Read the model definition and answer for the solid it produces. Units are mm, in the model's axes. A direction names the side the tool comes from. Give positions to 0.01 mm unless a question says otherwise; leave off trailing zeros. Order: outer loops, then holes, each group sorted by start corner. A loop starts at its lowest first (then second) coordinate and runs counter-clockwise, first axis right, second up.
```python
from build123d import *

# Parameters (mm, degrees)
F1_DEPTH = 20
F2_W     = 33
F2_H     = 34
F3_DEPTH = 39.001
F4_DEPTH = 6
F5_W     = 7.814886
F5_H     = 15.629771
F6_DEPTH = 25
F7_W     = 19.637413
F7_H     = 8.21565
F8_DEPTH = 39.001


with BuildPart() as f1:
    # F0 (on Front) → F1 (new body, symmetric)
    with BuildSketch(Plane.XZ):
        Polygon((0, 39), (0, 0), (39, 0), (39, 7), (7, 39), align=None)
    extrude(amount=F1_DEPTH, both=True)

    # F2 (on Top) → F3 (cut, through all)
    with BuildSketch(Plane.XY):
        with Locations((22.5, 0)):
            Rectangle(F2_W, F2_H)
    extrude(amount=F3_DEPTH, mode=Mode.SUBTRACT)

    # F2 (on Top) → F4 (join)
    with BuildSketch(Plane.XY):
        with Locations((22.5, 0)):
            Rectangle(F2_W, F2_H)
    extrude(amount=F4_DEPTH)

    # F5 (on face) → F6 (cut)
    with BuildSketch(Plane.YZ.offset(6)):
        with Locations((0, 22.542938)):
            Rectangle(F5_W, F5_H)
    extrude(amount=-F6_DEPTH, mode=Mode.SUBTRACT)

    # F7 (on Top) → F8 (cut, through all)
    with BuildSketch(Plane.XY):
        with Locations((22.542938, 0)):
            Rectangle(F7_W, F7_H)
    extrude(amount=F8_DEPTH, mode=Mode.SUBTRACT)


solid = f1.part
```
1) Given pin 1 (3 mm diameter, centred on y = 1.5, z = 4, fed in from -X); pin 2 (10 mm diameter, centred on x = 20, y = 8, fed in from +Z), each flat-ended and moving along its own axis, determine where each tip first touches the part or whether it passes through.
Final values:
pin 1: stops at x = 0
pin 2: stops at z = 6
2) For a pull along Y with two mould halves and no side action, classify faces 4 (the face through (15, 20, 15)), 5 (the face through (19, 17, 19)), 6 (the face through (15, -20, 15)) as released by +Y, released by -Y, zero draft, split by the parting line, or undercut.
Final values:
face 4: released by +Y
face 5: undercut
face 6: released by -Y
3) A tool of negligible diameter and unlimited length cuts with its end or side. For faces 1 (the face through (3, 0, 14.728)), 2 (the face through (19, -17, 19)), 3 (the face through (22, 4.108, 3)), from which of +Z, -Z, +X, -X, +Y, -Y can it reach the whole face along a straight path? Write none if from no direction.
Final values:
face 1: +X, -X
face 2: +Z, +X
face 3: +Z, -Z
4) The part is cut by section C-C on x = 11.5. Determine the outline of the cut face in (y, z), and give its area (3 significant figures).
Final values:
outline: (-20, 0) - (20, 0) - (20, 34.5) - (17, 34.5) - (17, 6) - (-17, 6) - (-17, 34.5) - (-20, 34.5) - close
area: 411 mm2
5) The part is cut by section A-A on x = 16.5. Determine the outline of the cut face in (y, z), and give its area (3 significant figures).
Final values:
outline: (-20, 0) - (-4.11, 0) - (-4.11, 6) - (-17, 6) - (-17, 29.5) - (-20, 29.5) - close; (4.11, 0) - (20, 0) - (20, 29.5) - (17, 29.5) - (17, 6) - (4.11, 6) - close
area: 332 mm2
6) The part is cut by section D-D on z = 4. Determine the outline of the cut face in (x, y), and give its area (3 significant figures).
Final values:
outline: (0, -20) - (39, -20) - (39, 20) - (0, 20) - close; hole (12.72, -4.11) - (32.36, -4.11) - (32.36, 4.11) - (12.72, 4.11) - close
area: 1,400 mm2
7) The part is cut by section B-B on z = 15.5. Determine the outline of the cut face in (x, y).
Final values:
outline: (0, -20) - (30.5, -20) - (30.5, -17) - (6, -17) - (6, -3.91) - (0, -3.91) - close; (0, 3.91) - (6, 3.91) - (6, 17) - (30.5, 17) - (30.5, 20) - (0, 20) - close
8) Consider L1, parallel to Y at x = 21, z = 16.5; L2, parallel to Y at x = 32, z = 3; L3, parallel to Z at x = 30, y = -13.5. Determine where each line is inside the solid, lowest interval first.
Final values:
L1: y = -20 to -17, 17 to 20
L2: y = -20 to -4.11, 4.11 to 20
L3: z = 0 to 6
